For this review, take the finished solid that the model builds, in its own axes (mm). A direction names the side the tool comes from. Give positions to 0.01 mm unless a question says otherwise; leave off trailing zeros. Write each loop counter-clockwise with the first axis right and the second up, starting at its lowest first coordinate (ties: lowest second). Pieces come first, ordered by that corner, then holes.
Q1. We need section C-C (z = 0). Give the number of separate pieces and of enclosed holes in the cut face, then the cut area to 3 significant figures.
Q2. We need section D-D (y = -7). Write out the cut boundary in (x, z).
Q3. Mouldability with a two-part tool opening along Y and no side actions: class faces 3 (the flat face through (-1, -38.1, 9)), 4 (the cylindrical face through (-34.687, 36.664, 0.511)), 5 (the cylindrical face through (-35.68, 28.94, 0.46)), 6 (the cylindrical face through (24.94, -35.68, 21.86)) as released by +Y, released by -Y, zero draft, split by the parting line, or undercut.
Q4. Machinability: for faces 1 (the flat face through (-33.325, 8, 1)), 2 (the cylindrical face through (-35.68, 28.94, 25.86)), which of the approach directions +Z, -Z, +X, -X, +Y, -Y give a long, thin tool a straight path to every point of the face, cutting with its end or side? Answer none if there is none.
Q5. For line 1 (Z direction, x = -25, y = -36); line 2 (X direction, y = -35.4, z = 25.4); line 3 (X direction, y = -34.95, z = 25.4), list the stretches that pass through material, from the lowest coordinate up.
Q6. Insertion check: P1, Ø5, axis at x = -26.5, z = 0.5, coming from the -Y side; P2, Ø11.5, axis at x = 25.4, z = 25.4, coming from the +Y side; P3, Ø12, axis at y = -1, z = -3.5, coming from the +X side; P4, Ø6.5, axis at y = 25.4, z = 25.4, coming from the -X side. Each pin has a flat end and moves straight along its axis. Give the tip position at first contact, or say it passes through.
Q7. We need section A-A (y = 25.4). Write out the cut boundary in (x, z).
```python
from build123d import *

# Parameters (mm, degrees)
BOSS_EXTRUDE1_DEPTH      = 36.5125
BOSS_EXTRUDE1_DEPTH_BACK = 36.5125
SKETCH4_R                = 3.5687
CUT_EXTRUDE1_DEPTH       = 5.7752
SKETCH5_R                = 3.5687
CUT_EXTRUDE2_DEPTH       = 5.7752


with BuildPart() as part:
    # Sketch3 → Boss-Extrude1 (new body, two sides)
    with BuildSketch(Plane.XY) as boss_extrude1_sk:
        with BuildLine():
            Line((-38.1, 38.1), (-38.1, -38.1))
            Line((-38.1, -38.1), (38.1, -38.1))
            ThreePointArc((38.1, -38.1), (36.701376302, -34.723423698), (33.3248, -33.3248))
            Line((33.3248, -33.3248), (-30.1498, -33.3248))
            ThreePointArc((-30.1498, -33.3248), (-32.39486403, -32.39486403), (-33.3248, -30.1498))
            Line((-33.3248, -30.1498), (-33.3248, 33.3248))
            ThreePointArc((-33.3248, 33.3248), (-34.723423698, 36.701376302), (-38.1, 38.1))
        make_face()
    extrude(amount=BOSS_EXTRUDE1_DEPTH)
    extrude(boss_extrude1_sk.sketch, amount=-BOSS_EXTRUDE1_DEPTH_BACK)

    # Sketch4 → Cut-Extrude1 (cut, through all)
    with BuildSketch(Plane(origin=(-33.3248, 0, 0), x_dir=(0, 0, -1), z_dir=(1, 0, 0))):
        with Locations((-25.4, -25.4)):
            Circle(SKETCH4_R)
        with Locations((0, -25.4)):
            Circle(SKETCH4_R)
        with Locations((25.4, -25.4)):
            Circle(SKETCH4_R)
        Circle(SKETCH4_R)
        with Locations((25.4, 0)):
            Circle(SKETCH4_R)
        with Locations((0, 25.4)):
            Circle(SKETCH4_R)
        with Locations((25.4, 25.4)):
            Circle(SKETCH4_R)
        with Locations((-25.4, 0)):
            Circle(SKETCH4_R)
        with Locations((-25.4, 25.4)):
            Circle(SKETCH4_R)
    extrude(amount=-CUT_EXTRUDE1_DEPTH, mode=Mode.SUBTRACT)

    # Sketch5 → Cut-Extrude2 (cut, through all)
    with BuildSketch(Plane(origin=(0, -33.3248, -33.3248), x_dir=(1, 0, 0), z_dir=(0, 1, 0))):
        with Locations((-25.4, -58.7248)):
            Circle(SKETCH5_R)
        with Locations((0, -58.7248)):
            Circle(SKETCH5_R)
        with Locations((25.4, -58.7248)):
            Circle(SKETCH5_R)
        with Locations((0, -33.3248)):
            Circle(SKETCH5_R)
        with Locations((25.4, -33.3248)):
            Circle(SKETCH5_R)
        with Locations((0, -7.9248)):
            Circle(SKETCH5_R)
        with Locations((25.4, -7.9248)):
            Circle(SKETCH5_R)
        with Locations((-25.4, -33.3248)):
            Circle(SKETCH5_R)
        with Locations((-25.4, -7.9248)):
            Circle(SKETCH5_R)
    extrude(amount=-CUT_EXTRUDE2_DEPTH, mode=Mode.SUBTRACT)


solid = part.part
```
Computed:
1. separate pieces: 7
1. enclosed holes: 0
1. area: 493 mm2
2. outline: (-38.1, -36.51) - (-33.32, -36.51) - (-33.32, 36.51) - (-38.1, 36.51) - close
3. face 3: released by -Y
3. face 4: released by +Y
3. face 5: undercut
3. face 6: zero draft
4. face 1: +Z, -Z, +X, +Y
4. face 2: +X, -X
5. line 1: z = -36.51 to -28.95, -21.85 to -3.55, 3.55 to 21.85, 28.95 to 36.51
5. line 2: x = -38.1 to -28.97, -21.83 to -3.57, 3.57 to 21.83, 28.97 to 37.26
5. line 3: x = -38.1 to -28.97, -21.83 to -3.57, 3.57 to 21.83, 28.97 to 36.91
6. P1: stops at y = -38.1
6. P2: stops at y = -33.32
6. P3: stops at x = -33.32
6. P4: passes through
7. outline: (-38.1, -36.51) - (-33.32, -36.51) - (-33.32, -28.97) - (-38.1, -28.97) - close; (-38.1, -21.83) - (-33.32, -21.83) - (-33.32, -3.57) - (-38.1, -3.57) - close; (-38.1, 3.57) - (-33.32, 3.57) - (-33.32, 21.83) - (-38.1, 21.83) - close; (-38.1, 28.97) - (-33.32, 28.97) - (-33.32, 36.51) - (-38.1, 36.51) - close
